Geometry check sheet. Reference: the model listing, model coordinates, mm. A direction names the side the tool comes from. Coordinates: 2 decimals unless noted, no trailing zeros. Write each loop counter-clockwise with the first axis right and the second up, starting at its lowest first coordinate (ties: lowest second). Pieces come first, ordered by that corner, then holes. Notation, with made-up numbers: (9, 74) -> (56, 74) arc R19 ccw to (56, 94) -> close; hole circle Ø8 at (25.25, -37.5). An arc over 180 degrees is marked (long way). Use a Markdown table: item, result.
```python
from build123d import *

# Parameters (mm, degrees)
BOSS_EXTRUDE1_DEPTH      = 30.3
BOSS_EXTRUDE1_DEPTH_BACK = 9.5
SKETCH4_R                = 0.8


with BuildPart() as part:
    # Sketch1 → Boss-Extrude1 (new, two sides: drawn at the far end of the back side and taken through both)
    with BuildSketch(Plane(origin=(0, 0, 0), x_dir=(1, 0, 0), z_dir=(0, 1, 0)).offset(-BOSS_EXTRUDE1_DEPTH_BACK)):
        Polygon((0.170807804, -2.864144671), (-2.863407818, 0.182744818), (-0.170807804, 2.864144671), (2.863407818, -0.182744818), align=None)
    extrude(amount=BOSS_EXTRUDE1_DEPTH + BOSS_EXTRUDE1_DEPTH_BACK)

    # Cut-Sweep1: sweep along a path in Sketch2
    with BuildLine(Plane(origin=(0, 0, 0), x_dir=(0.7056315400669045, 0, 0.7085789509030087), z_dir=(-0.7085789509030087, 0, 0.7056315400669045))) as cut_sweep1_path:
        Line((0, -9.5), (0, 20.2))
        ThreePointArc((0, 20.2), (-0.527207794, 21.472792206), (-1.8, 22))
        Line((-1.8, 22), (-2.25, 22))
    # Sketch4 → Cut-Sweep1 (sweep, cut)
    with BuildSketch(Plane.XZ.offset(9.5)):
        Circle(SKETCH4_R)
    sweep(path=cut_sweep1_path.line, mode=Mode.SUBTRACT)


solid = part.part
```
Item 1: Tool access check on faces 1 (the flat face through (1.325, 10.121, -1.362)), 2 (the cylindrical face through (-0.63, 5.56, 0.49)). Record the directions out of +Z, -Z, +X, -X, +Y, -Y that give a thin tool (end or side, any length) a straight path to the whole face; none if there is none.
Answer block:
| item | result |
|---|---|
| face 1 | -Z, +X, +Y, -Y |
| face 2 | -Y |
Item 2: Mould release check, pull along Y, two halves, no side actions. Record for faces 3 (the flat face through (1.54, 10.12, 1.5)), 4 (the flat face through (0, 30.3, 0)), 5 (the cylindrical face through (-1.4, 21.2, -1.4)): +Y half, -Y half, draft (parallel to the pull), parting line (faces both ways), or undercut.
Answer block:
| item | result |
|---|---|
| face 3 | draft |
| face 4 | +Y half |
| face 5 | undercut |
Item 3: Section check B-B on z = 1.55. Record the boundary of the cut face in (x, y).
Answer block:
| item | result |
|---|---|
| outline | (-1.14, -9.5) -> (1.49, -9.5) -> (1.49, 30.3) -> (-1.14, 30.3) -> close |
Item 4: Thickness scan on L1, parallel to Z at x = 0, y = 6.5; L2, parallel to X at y = 17.5, z = -0.1; L3, parallel to X at y = 21, z = 0.15. Record the ranges inside material, lowest first. Write a range as [from, to].
Answer block:
| item | result |
|---|---|
| L1 | z = [-2.69, -0.8], [0.8, 2.69] |
| L2 | x = [-2.78, -0.79], [0.79, 2.58] |
| L3 | x = [-2.53, -0.9], [0.67, 2.83] |
Item 5: Depth check by flat-ended pin: P1, Ø2, axis at y = -5.5, z = -2, coming from the +X side; P2, Ø1.5, axis at x = -1, z = 2, coming from the +Y side. Enter the tip coordinate at first touch or a pass-through.
Answer block:
| item | result |
|---|---|
| P1 | stops at x = 1.69 |
| P2 | stops at y = 30.3 |
Item 6: Section check A-A on y = 9.5. Record the boundary of the cut face in (x, z).
Answer block:
| item | result |
|---|---|
| outline | (-2.86, -0.18) -> (-0.17, -2.86) -> (2.86, 0.18) -> (0.17, 2.86) -> close; hole circle Ø1.6 at (0, 0) |
